Geometry: final body of the model. Coordinates: model frame, mm. Face numbers are marked on the shaded views. A direction names the side the tool comes from. Coordinates: 2 decimals unless noted, no trailing zeros. Order: outer loops, then holes, each group sorted by start corner. A loop starts at its lowest first (then second) coordinate and runs counter-clockwise, first axis right, second up. Notation, with made-up numbers: M 36,-35 L 66,-35 A18 cw 66,-27 Z; hole C 81,66.25 d9. An arc over 180 degrees is marked long. Use CSV: the item, a comma, the result in double quotes. Start each with the question number.
1. First-contact query: P1, Ø1, axis at y = 42, z = -4, coming from the +X side; P2, Ø2, axis at x = -78, y = 42, coming from the -Z side. Flat tips, straight axial feed; report the tip coordinate or a pass-through.
2. Section query C-C on z = -4.75. Return the cut outline in (x, y), and give its area (3 significant figures).
3. Set-up query: the marked faces 1 and 2. Return all of +Z, -Z, +X, -X, +Y, -Y with unobstructed straight access to the full face (end or side cutting, diameter ignored); none if empty.
4. Section query A-A on y = 39. Return the cut outline in (x, z).
5. Section query D-D on x = -52.5. Return the cut outline in (y, z).
6. Material intervals for line 1 (X direction, y = 38.75, z = 0.75); line 2 (X direction, y = 40.25, z = -6); line 3 (Z direction, x = -58, y = 36.5), sorted ascending.
7. Section query B-B on y = 36. Return the cut outline in (x, z), and give its area (3 significant figures).
from build123d import *

# Parameters (mm, degrees)
SKETCH2_W           = 75
SKETCH2_H           = 11.5
BOSS_EXTRUDE1_DEPTH = 2
SKETCH3_W           = 2
SKETCH3_H           = 11.5
BOSS_EXTRUDE2_DEPTH = 7
SKETCH4_W           = 2.5
SKETCH4_H           = 6.5
CUT_EXTRUDE1_DEPTH  = 10


with BuildPart() as part:
    # Sketch2 → Boss-Extrude1 (new body)
    with BuildSketch(Plane.XY):
        with Locations((-52.326839827, 40.245670996)):
            Rectangle(SKETCH2_W, SKETCH2_H)
    extrude(amount=BOSS_EXTRUDE1_DEPTH)

    # Sketch3 → Boss-Extrude2 (add)
    with BuildSketch(Plane(origin=(0, 0, 0), x_dir=(-1, 0, 0), z_dir=(0, 0, -1))):
        with Locations((88.826839827, 40.245670996)):
            Rectangle(SKETCH3_W, SKETCH3_H)
    extrude(amount=BOSS_EXTRUDE2_DEPTH)

    # Sketch4 → Cut-Extrude1 (cut)
    with BuildSketch(Plane.XY.offset(2)):
        with Locations((-19.076839827, 40.245670996)):
            Rectangle(SKETCH4_W, SKETCH4_H)
    extrude(amount=-CUT_EXTRUDE1_DEPTH, mode=Mode.SUBTRACT)


solid = part.part
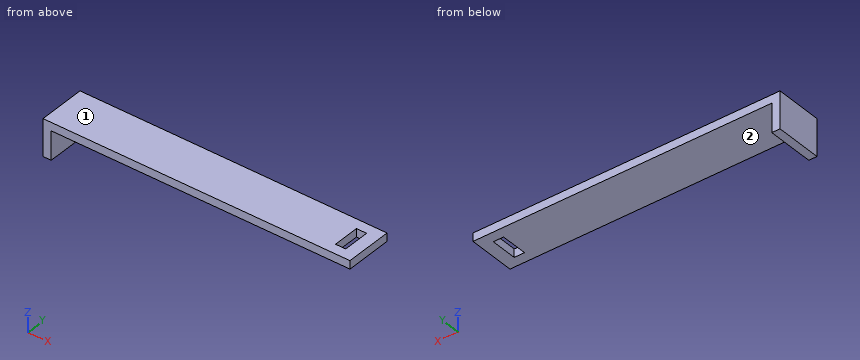
Results list:
1,P1,"stops at x = -87.83"
1,P2,"stops at z = 0"
2,outline,"M -89.83,34.5 L -87.83,34.5 L -87.83,46 L -89.83,46 Z"
2,area,"23.0 mm²"
3,face 1,"+Z, +X, -X, +Y, -Y"
3,face 2,"-Z, +X, +Y, -Y"
4,outline,"M -89.83,-7 L -87.83,-7 L -87.83,0 L -20.33,0 L -20.33,2 L -89.83,2 Z; M -17.83,0 L -14.83,0 L -14.83,2 L -17.83,2 Z"
5,outline,"M 34.5,0 L 46,0 L 46,2 L 34.5,2 Z"
6,line 1,"x = -89.83 to -20.33, -17.83 to -14.83"
6,line 2,"x = -89.83 to -87.83"
6,line 3,"z = 0 to 2"
7,outline,"M -89.83,-7 L -87.83,-7 L -87.83,0 L -14.83,0 L -14.83,2 L -89.83,2 Z"
7,area,"164 mm²"
